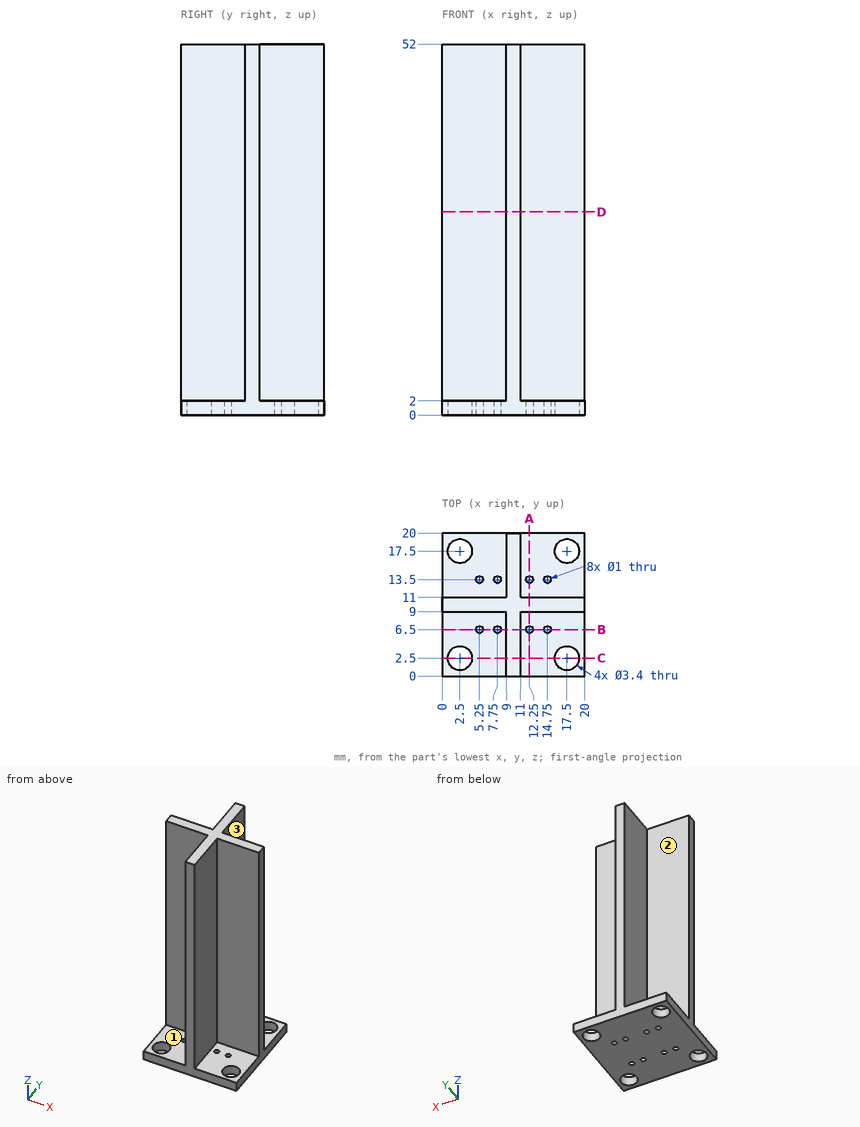
Design review of the part shown in the three views and the two pictorial views. Dimensions are in mm from the part's minimum x, y and z. A direction names the side the tool comes from. Round coordinates to 2 decimals unless told otherwise and drop trailing zeros. Write each loop counter-clockwise with the first axis right and the second up, starting at its lowest first coordinate (ties: lowest second). Pieces come first, ordered by that corner, then holes. Notation, with made-up numbers: M 66,9.25 L 95,9.25 A25 ccw 95,31.25 Z; hole C 68.25,-10.75 d10. An arc over 180 degrees is marked long. Use a Markdown table: item, result. Add a question column.
Q1. Machinability: for the marked faces 1, 2 and 3, which of the approach directions +Z, -Z, +X, -X, +Y, -Y give a long, thin tool a straight path to every point of the face, cutting with its end or side? Answer none if there is none.
Q2. Insertion check: pin 1 (7 mm diameter, centred on x = 15, y = 17, fed in from +Z); pin 2 (2.5 mm diameter, centred on x = 17.5, y = 2.5, fed in from +Z); pin 3 (2.5 mm diameter, centred on y = 5, z = 35.5, fed in from -X); pin 4 (2.5 mm diameter, centred on x = 6.5, z = 20, fed in from -Y). Each pin has a flat end and moves straight along its axis. Give the tip position at first contact, or say it passes through.
Q3. We need section B-B, the plane y = 6.5. State the section outline as (x, z) points.
Q4. We need section D-D, the plane z = 28.5. State the section outline as (x, y) points.
Q5. We need section C-C, the plane y = 2.5. State the section outline as (x, z) points.
Q6. To check wall thickness, follow line 1 (Y direction, x = 12.25, z = 1.5); line 2 (Y direction, x = 17.5, z = 0.9); line 3 (Y direction, x = 16.5, z = 15). State the ranges of each line that lie inside material, in increasing order.
Q7. We need section A-A, the plane x = 12.25. State the section outline as (y, z) points, plus the area to 3 significant figures.
Findings below:
| question | item | result |
|---|---|---|
| 1 | face 1 | +Z, -X, -Y |
| 1 | face 2 | +Z, -X, +Y |
| 1 | face 3 | +Z, +X, +Y |
| 2 | pin 1 | stops at z = 2 |
| 2 | pin 2 | passes through |
| 2 | pin 3 | stops at x = 9 |
| 2 | pin 4 | stops at y = 9 |
| 3 | outline | M 0,0 L 4.75,0 L 4.75,2 L 0,2 Z; M 5.75,0 L 7.25,0 L 7.25,2 L 5.75,2 Z; M 8.25,0 L 11.75,0 L 11.75,2 L 11,2 L 11,52 L 9,52 L 9,2 L 8.25,2 Z; M 12.75,0 L 14.25,0 L 14.25,2 L 12.75,2 Z; M 15.25,0 L 20,0 L 20,2 L 15.25,2 Z |
| 4 | outline | M 0,9 L 9,9 L 9,0 L 11,0 L 11,9 L 20,9 L 20,11 L 11,11 L 11,20 L 9,20 L 9,11 L 0,11 Z |
| 5 | outline | M 0,0 L 0.8,0 L 0.8,2 L 0,2 Z; M 4.2,0 L 15.8,0 L 15.8,2 L 11,2 L 11,52 L 9,52 L 9,2 L 4.2,2 Z; M 19.2,0 L 20,0 L 20,2 L 19.2,2 Z |
| 6 | line 1 | y = 0 to 6, 7 to 13, 14 to 20 |
| 6 | line 2 | y = 0 to 0.8, 4.2 to 15.8, 19.2 to 20 |
| 6 | line 3 | y = 9 to 11 |
| 7 | outline | M 0,0 L 6,0 L 6,2 L 0,2 Z; M 7,0 L 13,0 L 13,2 L 11,2 L 11,52 L 9,52 L 9,2 L 7,2 Z; M 14,0 L 20,0 L 20,2 L 14,2 Z |
| 7 | area | 136 mm² |
